```python
from build123d import *

# Parameters (mm, degrees)
EXTRUDE_1_DEPTH          = 120
CUT_EXTRUDE_1_DEPTH      = 34
CUT_EXTRUDE_1_DEPTH_BACK = 21
SKETCH_3_R               = 10


with BuildPart() as part:
    # 草图2 → 凸台-拉伸1 (new body)
    with BuildSketch(Plane(origin=(0, 0, 0), x_dir=(0, 0, -1), z_dir=(1, 0, 0))):
        Polygon((0, 0), (181.86, 0), (181.86, 5), (5, 5), (5, 130), (0, 130), align=None)
    extrude(amount=EXTRUDE_1_DEPTH)

    # 草图3 → 切除-拉伸1 (cut, two sides: drawn at the far end of the back side and taken through both)
    with BuildSketch(Plane.XY.offset(-CUT_EXTRUDE_1_DEPTH_BACK)):
        with Locations(Location((60, 65, 0), (0, 0, 270))):
            Circle(SKETCH_3_R)
    extrude(amount=CUT_EXTRUDE_1_DEPTH + CUT_EXTRUDE_1_DEPTH_BACK, mode=Mode.SUBTRACT)


solid = part.part
```
Source: CAD feature listing. Evaluate the final solid. Frame: model axes, mm. A direction names the side the tool comes from. Coordinates: 2 decimals unless noted, no trailing zeros. Loops run counter-clockwise (first coordinate to the right, second up) from the corner with the lowest first, then second, coordinate; pieces in that order, holes last. Notation, with made-up numbers: M 75.25,49.25 L 99.25,49.25 A15 cw 99.25,71.25 Z; hole C -33.5,49.5 d4. An arc over 180 degrees is marked long. Put each result on its own line as item: value. Start each with the question number.
1) Reachability of faces 5 (the face through (59, 130, -3)), 6 (the face through (46, 67, -5)) from +Z, -Z, +X, -X, +Y, -Y: full face, straight path, thin tool, end or side. Return the list, or none.
2) Cut plane B-B on x = 60. Return the cut outline in (y, z), then the cut area to 3 significant figures.
3) Pull-direction query (X, two-part tool) for faces 1 (the face through (54, 73, -3)), 2 (the face through (120, 3, -50)), 3 (the face through (0, 3, -50)), 4 (the face through (46, 66, 0)); classes: pulls with the +X half, pulls with the -X half, needs draft (parallel to the pull), parting line crosses it, or undercut.
4) Cut plane D-D on y = 25. Return the cut outline in (x, z).
5) Contact query for a flat-ended pin moving along its axis: pin 1 Ø8 at (x, y) = (69.5, 87) entering from -Z. Output: stop coordinate, or through.
6) Cut plane A-A on y = 65. Return the cut outline in (x, z), then the cut area to 3 significant figures.
7) Ray query, L1, parallel to Y at x = 60, z = -2; L2, parallel to X at y = 65, z = -2.9; L3, parallel to Z at x = 24, y = 107.5. Return the intervals inside material, ascending. Write a range as from..to.
8) Cut plane C-C on x = 45. Return the cut outline in (y, z).
The answers:
1. face 5: +Z, -Z, +X, -X, +Y
1. face 6: -Z, +X, -X, +Y
2. outline: M 0,-181.86 L 5,-181.86 L 5,-5 L 55,-5 L 55,0 L 0,0 Z; M 75,-5 L 130,-5 L 130,0 L 75,0 Z
2. area: 1,430 mm²
3. face 1: undercut
3. face 2: pulls with the +X half
3. face 3: pulls with the -X half
3. face 4: needs draft
4. outline: M 0,-5 L 120,-5 L 120,0 L 0,0 Z
5. pin 1: stops at z = -5
6. outline: M 0,-5 L 50,-5 L 50,0 L 0,0 Z; M 70,-5 L 120,-5 L 120,0 L 70,0 Z
6. area: 500 mm²
7. L1: y = 0..55, 75..130
7. L2: x = 0..50, 70..120
7. L3: z = -5..0
8. outline: M 0,-181.86 L 5,-181.86 L 5,-5 L 130,-5 L 130,0 L 0,0 Z
